from build123d import *
from OCP.BRepAlgoAPI import BRepAlgoAPI_Cut
from OCP.TopTools import TopTools_ListOfShape

# Parameters (mm, degrees)
SKETCH_1_R          = 11.15
SKETCH_1_R_2        = 1.5
EXTRUDE_1_DEPTH     = 5
SKETCH_2_W          = 14
SKETCH_2_H          = 10
SKETCH_2_W_2        = 15
SKETCH_2_W_3        = 5
SKETCH_2_H_2        = 5
EXTRUDE_2_DEPTH     = 5
SKETCH_2_3_W        = 14
SKETCH_2_3_H        = 7.3
EXTRUDE_6_DEPTH     = 25
SKETCH_6_W          = 14
SKETCH_6_H          = 7.3
EXTRUDE_7_DEPTH     = 5
SKETCH_7_W          = 67.3
SKETCH_7_H          = 34
EXTRUDE_8_DEPTH     = 5
FILLET_9_R          = 3.5
FILLET_8_R          = 1
FILLET_10_DEPTH     = 4.450151431
FILLET_START        = 4.450151431
FILLET_10_2_DEPTH   = 0.549848569
FILLET_START_2      = 19.24183889
FILLET_10_3_DEPTH   = 1.90816111
FILLET_11_R         = 3.5
SKETCH_8_R          = 2.5
CUT_EXTRUDE_1_DEPTH = 5
SKETCH_9_R          = 2.5
CUT_EXTRUDE_2_DEPTH = 5
SKETCH_10_R         = 2.5
CUT_EXTRUDE_3_DEPTH = 5


with BuildPart() as part:
    # 스케치1 → 보스-돌출1 (new body)
    with BuildSketch(Plane.XY):
        Polygon((-21.15, -16.15), (-21.15, 16.15), (-16.15, 21.15), (16.15, 21.15), (21.15, 16.15), (21.15, -16.15), (16.15, -21.15), (-16.15, -21.15), align=None)
        Circle(SKETCH_1_R, mode=Mode.SUBTRACT)
        with Locations((15.5, 15.5)):
            Circle(SKETCH_1_R_2, mode=Mode.SUBTRACT)
        with Locations((-15.5, 15.5)):
            Circle(SKETCH_1_R_2, mode=Mode.SUBTRACT)
        with Locations((15.5, -15.5)):
            Circle(SKETCH_1_R_2, mode=Mode.SUBTRACT)
        with Locations((-15.5, -15.5)):
            Circle(SKETCH_1_R_2, mode=Mode.SUBTRACT)
    extrude(amount=EXTRUDE_1_DEPTH)

    # 스케치2 → 보스-돌출2 (add)
    with BuildSketch(Plane(origin=(21.15, 0, 0), x_dir=(0, 0, -1), z_dir=(1, 0, 0))):
        with Locations((22, 11.15)):
            Rectangle(SKETCH_2_W, SKETCH_2_H)
        with Locations((7.5, 11.15)):
            Rectangle(SKETCH_2_W_2, SKETCH_2_H)
        with Locations((-2.5, 11.15)):
            Rectangle(SKETCH_2_W_3, SKETCH_2_H)
        with Locations((-2.5, 18.65)):
            Rectangle(SKETCH_2_W_3, SKETCH_2_H_2)
        with Locations((7.5, 18.65)):
            Rectangle(SKETCH_2_W_2, SKETCH_2_H_2)
        with Locations((22, 18.65)):
            Rectangle(SKETCH_2_W, SKETCH_2_H_2)
    extrude(amount=EXTRUDE_2_DEPTH)

    # 스케치2<3> → 보스-돌출6 (add)
    with BuildSketch(Plane(origin=(21.15, 0, 0), x_dir=(0, 0, -1), z_dir=(1, 0, 0))):
        with Locations((22, 2.5)):
            Rectangle(SKETCH_2_3_W, SKETCH_2_3_H)
    extrude(amount=EXTRUDE_6_DEPTH)

    # 스케치6 → 보스-돌출7 (add)
    with BuildSketch(Plane(origin=(46.15, 0, 0), x_dir=(0, 0, -1), z_dir=(1, 0, 0))):
        with Locations((22, 2.5)):
            Rectangle(SKETCH_6_W, SKETCH_6_H)
        Polygon((15, -1.15), (15, 6.15), (-5, 6.15), (-5, -21.15), (29, -21.15), (29, -1.15), align=None)
    extrude(amount=EXTRUDE_7_DEPTH)

    # 스케치7 → 보스-돌출8 (add)
    with BuildSketch(Plane.XZ.offset(21.15)):
        with Locations((17.5, -12)):
            Rectangle(SKETCH_7_W, SKETCH_7_H)
    extrude(amount=EXTRUDE_8_DEPTH)

    # 필렛9
    # the kernel refuses this fillet: 3.5 mm, written as the material it adds along each edge
    with BuildSketch(Plane(origin=(16.15, -21.15, 0), x_dir=(1, 0, 0), z_dir=(0, 0, 1))) as fillet_9_piece_1:
        with BuildLine():
            CenterArc((8.16227766, 3.5), FILLET_9_R, 154.623066475, 115.376933525)
            Line((5, 5), (0, 0))
            Line((0, 0), (8.16227766, 0))
        make_face()
    extrude(amount=5)

    # 필렛8
    fillet_8_edges = [part.edges().sort_by_distance(p)[0] for p in [
        (17.5, -26.15, -29),
        (21.354237769, -19.520828693, 5),
        (21.15, 10, -29),
        (26.15, 21.15, -12),
        (23.65, 21.15, -29),
        (23.65, 21.15, 5),
        (26.15, 13.65, -29),
        (26.15, 13.65, 5),
        (36.15, 6.15, -15),
        (33.65, -1.15, -29),
        (38.65, 6.15, -29),
        (46.15, 6.15, -5),
        (46.15, -7.5, 5),
        (48.65, 6.15, 5),
        (46.15, -11.15, -29),
        (51.15, 6.15, -12),
        (51.15, -10, 5),
        (51.15, -10, -29),
        (35.23113883, -21.15, 5),
        (15, -21.15, -29),
        (-16.15, -23.65, -29),
        (51.15, -26.15, -12),
        (17.5, -26.15, 5),
        (-16.15, -26.15, -12),
    ]]
    fillet(fillet_8_edges, radius=FILLET_8_R)


with BuildPart() as fillet_10_tool:
    # 필렛10: read off the stored shape, not the designer's step
    # 필렛10 outline → 필렛10 (new body)
    with BuildSketch(Plane.XY):
        with BuildLine():
            ThreePointArc((21.150000872, 21.15000089), (18.667895356, 20.099665017), (16.175253817, 21.124746183))
            Line((16.175253817, 21.124746183), (21.15, 16.15))
            Line((21.15, 16.15), (21.150000872, 21.15000089))
        make_face()
    extrude(amount=FILLET_10_DEPTH)


with BuildPart() as part_1:
    add(part.part)


with BuildPart() as part_2:
    # 필렛10: joined with fillet_10_tool
    add(part_1.part.fuse(fillet_10_tool.part, tol=0.00001))


with BuildPart() as fillet_10_2_tool:
    # Fillet 10 2 outline → Fillet 10 2 (new body)
    with BuildSketch(Plane.XY.offset(FILLET_START)):
        with BuildLine():
            ThreePointArc((21.150000872, 21.15000089), (18.667895356, 20.099665017), (16.175253817, 21.124746183))
            Line((16.175253817, 21.124746183), (21.15, 16.15))
            Line((21.15, 16.15), (21.15, 21.042952232))
            Line((21.15, 21.042952232), (21.150000872, 21.15000089))
        make_face()
    extrude(amount=FILLET_10_2_DEPTH)


with BuildPart() as part_3:
    add(part_2.part)


with BuildPart() as part_4:
    # Fillet 10 2: joined with fillet_10_2_tool
    add(part_3.part.fuse(fillet_10_2_tool.part, tol=0.00001))


with BuildPart() as fillet_10_3_tool:
    # Fillet 10 3 outline → Fillet 10 3 (new body)
    with BuildSketch(Plane.YZ.offset(FILLET_START_2)):
        with BuildLine():
            Line((19, 5.000000001), (20.15, 5))
            ThreePointArc((20.15, 5), (20.857106781, 4.707106781), (21.15, 4))
            Line((21.15, 4), (21.150000003, -1))
            Line((21.150000003, -1), (23, -1))
            Line((23, -1), (23, 6))
            Line((23, 6), (19, 6))
            Line((19, 6), (19, 5.000000001))
        make_face()
    extrude(amount=FILLET_10_3_DEPTH)


with BuildPart() as part_5:
    add(part_4.part)

    # Fillet 10 3: cut by fillet_10_3_tool, with a tolerance
    fillet_10_3_stock = TopTools_ListOfShape()
    fillet_10_3_stock.Append(part_5.part.wrapped)
    fillet_10_3_tools = TopTools_ListOfShape()
    fillet_10_3_tools.Append(fillet_10_3_tool.part.wrapped)
    fillet_10_3_cut = BRepAlgoAPI_Cut()
    fillet_10_3_cut.SetArguments(fillet_10_3_stock)
    fillet_10_3_cut.SetTools(fillet_10_3_tools)
    fillet_10_3_cut.SetFuzzyValue(0.00001)
    fillet_10_3_cut.Build()
    add(Compound.cast(fillet_10_3_cut.Shape()).solids(), mode=Mode.REPLACE)

    # 필렛11
    # the kernel refuses this fillet: 3.5 mm, written as the material it takes off along each edge
    with BuildSketch(Plane(origin=(24.65, 2.35, -29), x_dir=(0, -1, 0), z_dir=(1, 0, 0))) as fillet_11_piece_1:
        with BuildLine():
            CenterArc((2.5, -1), 1, 0, 90)
            Line((3.5, -1), (3.5, 0))
            Line((3.5, 0), (2.5, 0))
        make_face()
    revolve(axis=Axis((24.65, 2.35, -29), (0, 0, -1)), revolution_arc=90, mode=Mode.SUBTRACT)
    with BuildSketch(Plane(origin=(24.65, 2.35, -18.5), x_dir=(-1, 0, 0), z_dir=(0, 0, 1))) as fillet_11_piece_2_section:
        Polygon((0, 0), (FILLET_11_R, 0), (FILLET_11_R, FILLET_11_R), (0, FILLET_11_R), align=None)
    fillet_11_piece_2 = extrude(amount=FILLET_11_R, mode=Mode.PRIVATE)
    fillet_11_piece_2 = fillet_11_piece_2 - Plane(origin=(24.65, 2.35, -18.5), x_dir=(0.7071067811865475, 0.7071067811865475, 0), z_dir=(0, 0, 1)) * Sphere(FILLET_11_R, mode=Mode.PRIVATE)
    add(fillet_11_piece_2, mode=Mode.SUBTRACT)
    with BuildSketch(Plane(origin=(21.15, 6.15, -15), x_dir=(1, 0, 0), z_dir=(0, -1, 0))) as fillet_11_piece_3:
        with BuildLine():
            CenterArc((FILLET_11_R, -FILLET_11_R), FILLET_11_R, 90, 90)
            Line((0, -FILLET_11_R), (0, 0))
            Line((0, 0), (FILLET_11_R, 0))
        make_face()
    extrude(amount=3.8, mode=Mode.SUBTRACT)
    with BuildSketch(Plane(origin=(21.15, -1.15, -18.5), x_dir=(0, 1, 0), z_dir=(0, 0, -1))) as fillet_11_piece_4:
        with BuildLine():
            CenterArc((FILLET_11_R, FILLET_11_R), FILLET_11_R, 180, 90)
            Line((0, FILLET_11_R), (0, 0))
            Line((0, 0), (FILLET_11_R, 0))
        make_face()
    extrude(amount=10.5, mode=Mode.SUBTRACT)
    with BuildSketch(Plane(origin=(24.65, -1.15, -15), x_dir=(0, 1, 0), z_dir=(1, 0, 0))) as fillet_11_piece_5:
        with BuildLine():
            CenterArc((FILLET_11_R, -FILLET_11_R), FILLET_11_R, 90, 90)
            Line((0, -FILLET_11_R), (0, 0))
            Line((0, 0), (FILLET_11_R, 0))
        make_face()
    extrude(amount=21.5, mode=Mode.SUBTRACT)

    # 스케치8 → 컷-돌출1 (cut)
    with BuildSketch(Plane(origin=(0, 6.15, 0), x_dir=(1, 0, 0), z_dir=(0, 1, 0))):
        with Locations(Location((36.65, 22, 0), (0, 0, 270))):
            Circle(SKETCH_8_R)
    extrude(amount=-CUT_EXTRUDE_1_DEPTH, mode=Mode.SUBTRACT)

    # 스케치9 → 컷-돌출2 (cut)
    with BuildSketch(Plane(origin=(51.15, 0, 0), x_dir=(0, 0, -1), z_dir=(1, 0, 0))):
        with Locations((4.5, -10)):
            Circle(SKETCH_9_R)
        with Locations((19.5, -10)):
            Circle(SKETCH_9_R)
    extrude(amount=-CUT_EXTRUDE_2_DEPTH, mode=Mode.SUBTRACT)

    # 스케치10 → 컷-돌출3 (cut)
    with BuildSketch(Plane(origin=(0, -21.15, 0), x_dir=(1, 0, 0), z_dir=(0, 1, 0))):
        with Locations(Location((36.65, 22, 0), (0, 0, 270))):
            Circle(SKETCH_10_R)
        with Locations(Location((36.65, 12, 0), (0, 0, 270))):
            Circle(SKETCH_10_R)
        with Locations(Location((36.65, 2, 0), (0, 0, 270))):
            Circle(SKETCH_10_R)
    extrude(amount=-CUT_EXTRUDE_3_DEPTH, mode=Mode.SUBTRACT)


solid = part_5.part
Work out the finished part from the listing and answer in its coordinate system (mm). A direction names the side the tool comes from. Coordinates: 2 decimals unless noted, no trailing zeros. Loops run counter-clockwise (first coordinate to the right, second up) from the corner with the lowest first, then second, coordinate; pieces in that order, holes last. Notation, with made-up numbers: M -26,11 L 28,11 A27 ccw 28,47 Z; hole C -19.75,66 d1. An arc over 180 degrees is marked long. Answer in a Markdown table with one row per item. Add a question column.
1. A tool of negligible diameter and unlimited length cuts with its end or side. For faces 5 (the flat face through (35, 4, -15)), 6 (the flat face through (41, 6.15, -19)), 7 (the flat face through (24, 6.15, -7)), from which of +Z, -Z, +X, -X, +Y, -Y can it reach the whole face along a straight path? Write none if from no direction.
2. Consider L1, parallel to X at y = 3, z = -22; L2, parallel to Y at x = 23, z = -8.5; L3, parallel to Y at x = 47.6, z = -19.5. Determine where each line is inside the solid, lowest interval first.
3. Find section B-B, the plane y = 10. Write down the section's boundary in (x, z).
4. The mould has two halves that part along Y. Classify faces 1 (the cylindrical face through (49, -12, -18)), 2 (the flat face through (35, -1.15, -23)), 3 (the flat face through (26.15, 13, -12)), 4 (the flat face through (37, 1.15, -22)): pulls with the +Y half, pulls with the -Y half, needs draft (parallel to the pull), parting line crosses it, or undercut.
5. Find section A-A, the plane x = -3.5. Write down the section's boundary in (y, z), then the cut area to 3 significant figures.
6. Flat-ended cylindrical pins translate along their axes: P1, Ø4.5, axis at y = -22.5, z = -16, coming from the -X side; P2, Ø12, axis at x = 9.5, z = -20.5, coming from the +Y side; P3, Ø2.5, axis at x = -15.5, y = -15.5, coming from the -Z side; P4, Ø6, axis at x = 29.5, z = -15, coming from the +Y side. Find the tip coordinate at first contact, or state that the pin passes through.
7. Find section C-C, the plane y = 18. Write down the section's boundary in (x, z), then the cut area to 3 significant figures.
Reported:
| question | item | result |
|---|---|---|
| 1 | face 5 | +Z, -X |
| 1 | face 6 | +Z, -Z, +X, +Y |
| 1 | face 7 | +Z |
| 2 | L1 | x = 21.15 to 34.15, 39.15 to 51.15 |
| 2 | L2 | y = -26.15 to -21.15, 6.15 to 21.15 |
| 2 | L3 | y = -26.15 to -12.5, -7.5 to 6.15 |
| 3 | outline | M -21.15,0 L -4.93,0 L -4.93,5 L -21.15,5 Z; M 4.93,0 L 21.15,0 L 21.15,-28 A1 ccw 22.15,-29 L 25.15,-29 A1 ccw 26.15,-28 L 26.15,4 A1 ccw 25.15,5 L 4.93,5 Z |
| 4 | face 1 | undercut |
| 4 | face 2 | undercut |
| 4 | face 3 | needs draft |
| 4 | face 4 | pulls with the +Y half |
| 5 | outline | M -26.15,-28 A1 ccw -25.15,-29 L -22.15,-29 A1 ccw -21.15,-28 L -21.15,0 L -10.59,0 L -10.59,5 L -25.15,5 A1 ccw -26.15,4 Z; M 10.59,0 L 21.15,0 L 21.15,5 L 10.59,5 Z |
| 5 | area | 275 mm^2 |
| 6 | P1 | stops at x = -16.15 |
| 6 | P2 | stops at y = -21.15 |
| 6 | P3 | passes through |
| 6 | P4 | stops at y = 6.15 |
| 7 | outline | M -19.3,0 L 21.15,0 L 21.15,-28 A1 ccw 22.15,-29 L 25.15,-29 A1 ccw 26.15,-28 L 26.15,4 A1 ccw 25.15,5 L -19.3,5 Z |
| 7 | area | 372 mm^2 |
